Could you check a few things on this drawing? It's one solid part, dimensions in mm from its lowest x, y, z. A direction names the side the tool comes from. Give positions to 0.01 mm unless a question says otherwise; leave off trailing zeros. Loops run counter-clockwise (first coordinate to the right, second up) from the corner with the lowest first, then second, coordinate; pieces in that order, holes last.
1. For P1, Ø1, axis at y = 15, z = 11, coming from the +X side; P2, Ø4.5, axis at x = 4.5, y = 15, coming from the -Z side (1 decimal); P3, Ø4.5, axis at x = 43.06, y = 24.41, coming from the +Z side, each with a flat end and sliding along its axis, tell me the tip position at first contact or that it passes through.
2. Imagine slicing it at B-B (y = 27). List the corners of the cut face in (x, z) for me (1 decimal).
3. Imagine slicing it at D-D (y = 18.5). List the corners of the cut face in (x, z) for me (1 decimal).
4. I need wall thicknesses on line 1 along X through (y, z) = (24.5, 6.5) (1 decimal); line 2 along X through (y, z) = (9.5, 9.25) (1 decimal); line 3 along Y through (x, z) = (36, 1.75). Which ranges of each line are inside material? Lowest first, please.
5. Thinking about a two-plate mould opening in Y: for the marked faces 4, 5, 6 and 7, which applies, +Y half, -Y half, draft (parallel to the pull), parting line (faces both ways), or undercut?
6. For the marked faces 1, 2 and 3, which set-ups out of +Z, -Z, +X, -X, +Y, -Y let a thin tool reach every point of the face, with its end or its side?
7. Imagine slicing it at C-C (x = 19). List the corners of the cut face in (y, z) for me.
8. Imagine slicing it at A-A (z = 12.75). List the corners of the cut face in (x, y) for me (1 decimal).
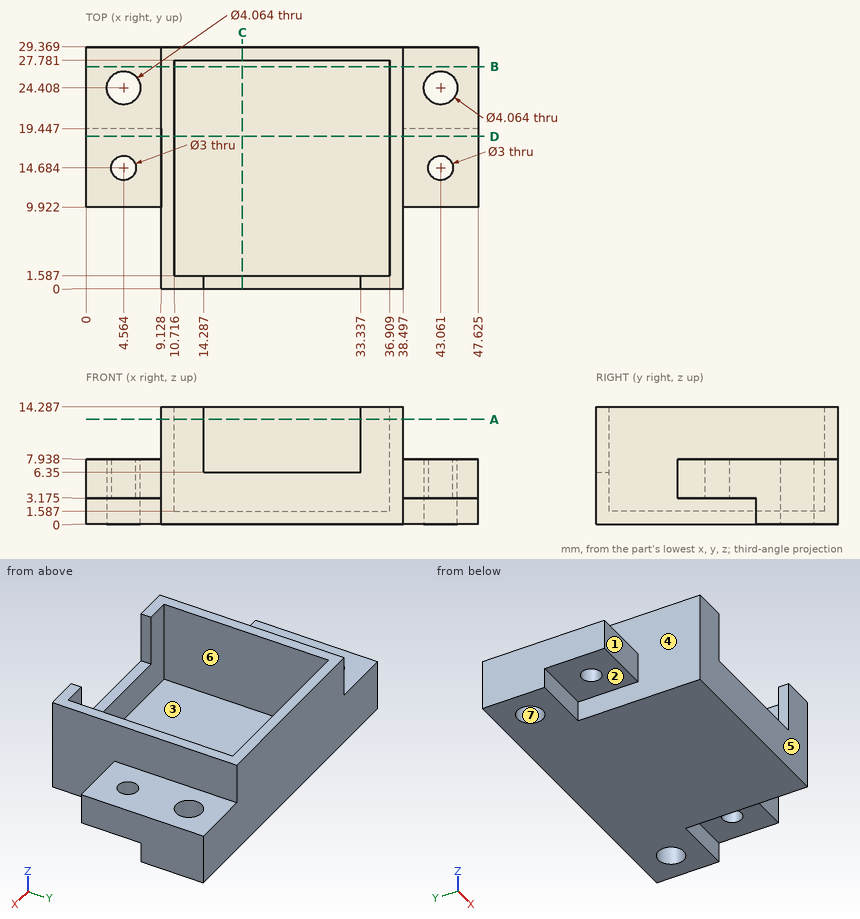
Derived:
1. P1: stops at x = 38.5
1. P2: stops at z = 3.2
1. P3: stops at z = 7.94
2. outline: (0, 0) - (47.6, 0) - (47.6, 7.9) - (38.5, 7.9) - (38.5, 14.3) - (36.9, 14.3) - (36.9, 1.6) - (10.7, 1.6) - (10.7, 14.3) - (9.1, 14.3) - (9.1, 7.9) - (0, 7.9) - close
3. outline: (0, 3.2) - (9.1, 3.2) - (9.1, 0) - (38.5, 0) - (38.5, 3.2) - (47.6, 3.2) - (47.6, 7.9) - (38.5, 7.9) - (38.5, 14.3) - (36.9, 14.3) - (36.9, 1.6) - (10.7, 1.6) - (10.7, 14.3) - (9.1, 14.3) - (9.1, 7.9) - (0, 7.9) - close
4. line 1: x = 0 to 2.5, 6.6 to 10.7, 36.9 to 41, 45.1 to 47.6
4. line 2: x = 9.1 to 10.7, 36.9 to 38.5
4. line 3: y = 0 to 1.59, 27.78 to 29.37
5. face 4: draft
5. face 5: -Y half
5. face 6: undercut
5. face 7: undercut
6. face 1: +Z, -Z, -X, -Y
6. face 2: -Z, -X, -Y
6. face 3: +Z
7. outline: (0, 0) - (29.37, 0) - (29.37, 14.29) - (27.78, 14.29) - (27.78, 1.59) - (1.59, 1.59) - (1.59, 6.35) - (0, 6.35) - close
8. outline: (9.1, 0) - (14.3, 0) - (14.3, 1.6) - (10.7, 1.6) - (10.7, 27.8) - (36.9, 27.8) - (36.9, 1.6) - (33.3, 1.6) - (33.3, 0) - (38.5, 0) - (38.5, 29.4) - (9.1, 29.4) - close
